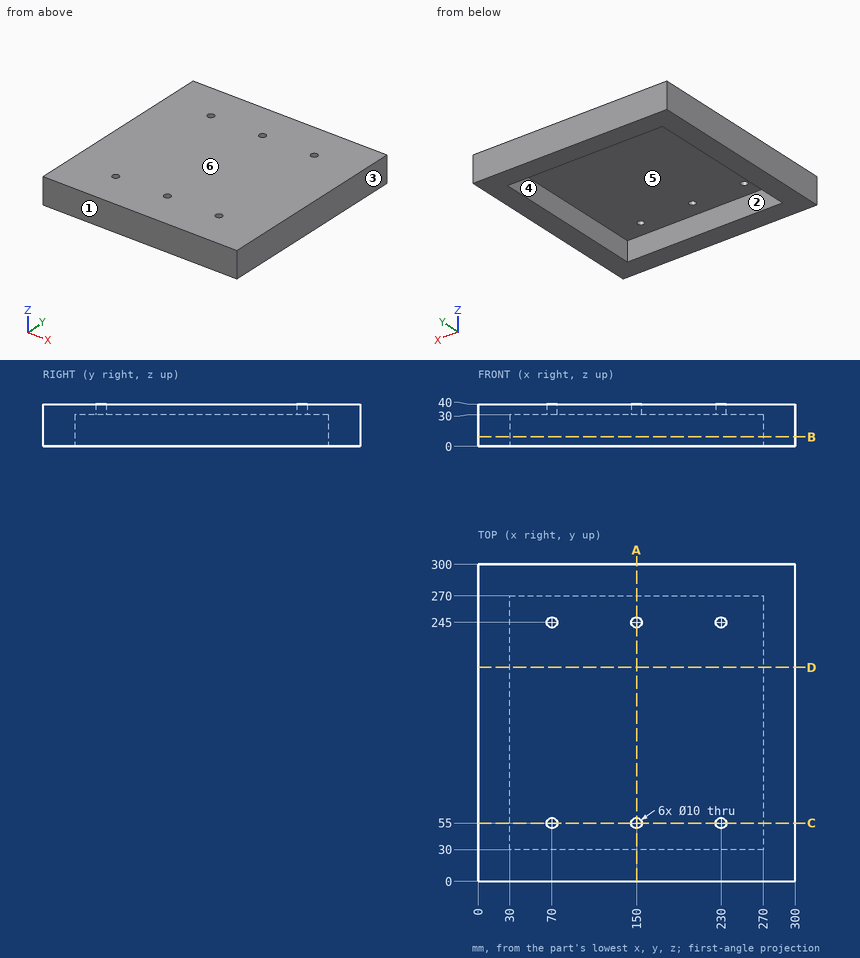
Study the drawing (mm; zero at the part's minimum x, y, z) and answer. A direction names the side the tool comes from. Coordinates: 2 decimals unless noted, no trailing zeros. Write each loop counter-clockwise with the first axis right and the second up, starting at its lowest first coordinate (ties: lowest second). Pieces come first, ordered by that corner, then holes.
Q1. Section C-C, the plane y = 55 is taken. Write down the section's boundary in (x, z), then the cut area to 3 significant figures.
Returned:
outline: (0, 0) - (30, 0) - (30, 30) - (65, 30) - (65, 40) - (0, 40) - close; (75, 30) - (145, 30) - (145, 40) - (75, 40) - close; (155, 30) - (225, 30) - (225, 40) - (155, 40) - close; (235, 30) - (270, 30) - (270, 0) - (300, 0) - (300, 40) - (235, 40) - close
area: 4,500 mm2
Q2. Section D-D, the plane y = 202.5 is taken. Write down the section's boundary in (x, z).
Returned:
outline: (0, 0) - (30, 0) - (30, 30) - (270, 30) - (270, 0) - (300, 0) - (300, 40) - (0, 40) - close
Q3. Section A-A, the plane x = 150 is taken. Write down the section's boundary in (y, z), then the cut area to 3 significant figures.
Returned:
outline: (0, 0) - (30, 0) - (30, 30) - (50, 30) - (50, 40) - (0, 40) - close; (60, 30) - (240, 30) - (240, 40) - (60, 40) - close; (250, 30) - (270, 30) - (270, 0) - (300, 0) - (300, 40) - (250, 40) - close
area: 4,600 mm2
Q4. Section B-B, the plane z = 9 is taken. Write down the section's boundary in (x, y).
Returned:
outline: (0, 0) - (300, 0) - (300, 300) - (0, 300) - close; hole (30, 30) - (270, 30) - (270, 270) - (30, 270) - close
Q5. The mould has two halves that part along X. Classify the marked faces 1, 2, 3 and 4: released by +X, released by -X, zero draft, split by the parting line, or undercut.
Returned:
face 1: zero draft
face 2: undercut
face 3: released by +X
face 4: undercut
Q6. Given P1, Ø16, axis at x = 150, y = 245, coming from the -Z side, flat-ended and moving along its own axis, determine where the tip first touches the part or whether it passes through.
Returned:
P1: stops at z = 30
Q7. Which of the six approach directions +Z, -Z, +X, -X, +Y, -Y give full straight-line access (tool end or side, diameter ignored) to the marked faces 5 and 6?
Returned:
face 5: -Z
face 6: +Z, +X, -X, +Y, -Y
Q8. Find the intervals of material crossed by line 1 along X through (y, z) = (245, 37); line 2 along Y through (x, z) = (230, 37); line 3 along X through (y, z) = (53.5, 29), in increasing order.
Returned:
line 1: x = 0 to 65, 75 to 145, 155 to 225, 235 to 300
line 2: y = 0 to 50, 60 to 240, 250 to 300
line 3: x = 0 to 30, 270 to 300
